Autodesk Inventor part; units mm, degrees
ref_plane "Work Plane2" through (17.8, 0, -35.7) normal (-1, 0, 0) x (0, 0, 1)
ref_plane "Work Plane3" through (20.6, 0, 2) normal (1, 0, 0) x (0, 0, -1)
ref_plane "YZ Plane" through (0, 0, 0) normal (1, 0, 0) x (0, 1, 0)
sketch "Sketch1" plane through (0, 0, 0) normal (0, 1, 0) x (-1, 0, 0)
  line L0 (0, 0) -> (-41.2, 0)
  line L1 (-41.2, 0) -> (-41.2, -33.7)
  line L2 (-41.2, -33.7) -> (0, -33.7)
  line L3 (0, -33.7) -> (0, 0)
  line L4 (2, 2) -> (-43.2, 2)
  line L5 (-43.2, 2) -> (-43.2, -35.7)
  line L6 (-43.2, -35.7) -> (2, -35.7)
  line L7 (2, -35.7) -> (2, 2)
  dimension "d0" = 33.7
  dimension "d1" = 41.2
  dimension "d2" = 2
  dimension "d3" = 2
  dimension "d4" = 2
  dimension "d5" = 2
extrude "Extrusion1" add sketch "Sketch1" along normal blind 2 contours L3 L2 L1 L0
extrude "Extrusion2" add sketch "Sketch1" along normal blind 120.5
sketch "Sketch2" plane through (41.2, 2, 0) normal (0, 0, -1) x (-1, 0, 0)
  line L0 (43.2, 118.5) -> (-2, 118.5)
  line L1 (36.2, 118.5) -> (31.2, 118.5)
  line L2 (31.2, 118.5) -> (31.2, 116.5)
  line L3 (31.2, 116.5) -> (36.2, 116.5)
  line L4 (36.2, 116.5) -> (36.2, 118.5)
  line L5 (41.2, 0) -> (41.2, 118.5)
  point P0 (41.2, -2)
  point P1 (31.2, 118.5)
  dimension "d10" = 5
  dimension "d11" = 2
  dimension "d12" = 5
sketch "Sketch3" plane through (41.2, 2, 0) normal (-1, 0, 0) x (0, 0, 1)
  point P0 (0, -2)
sketch "Sketch4" plane through (41.2, 2, 0) normal (-1, 0, 0) x (0, 0, 1)
  line L0 (2, 118.5) -> (-35.7, 118.5)
  line L1 (-5, 118.5) -> (-10, 118.5)
  line L2 (-10, 118.5) -> (-10, 116.5)
  line L3 (-10, 116.5) -> (-5, 116.5)
  line L4 (-5, 116.5) -> (-5, 118.5)
  line L5 (0, 0) -> (0, 118.5)
  point P0 (0, -2)
  dimension "d27" = 5
  dimension "d28" = 2
  dimension "d29" = 5
extrude "Extrusion4" add sketch "Sketch4" along normal blind 1.5
chamfer "Chamfer5" distance 0.75 distance2 1.5 1 edges at (39.7, 120.5, -7.5) measured on face at (39.7, 119.1667, -6.6667)
chamfer "Chamfer6" distance 0.75 distance2 1.5 1 edges at (39.7, 119.125, -10) measured on face at (39.7, 118.9167, -6.6667)
chamfer "Chamfer7" distance 0.75 distance2 1.5 1 edges at (39.7, 118.5, -7.1251) measured on face at (39.7, 119.3333, -7.8334)
chamfer "Chamfer8" distance 0.75 distance2 1.5 1 edges at (39.7, 119.5, -5) measured on face at (39.7, 119.5833, -6.4167)
sketch "Sketch5" plane through (0, 2, -33.7) normal (0, 0, 1) x (1, 0, 0)
  line L0 (0, 118.5) -> (41.2, 118.5)
  line L1 (36.2, 118.5) -> (31.2, 118.5)
  line L2 (31.2, 118.5) -> (31.2, 116.5)
  line L3 (31.2, 116.5) -> (36.2, 116.5)
  line L4 (36.2, 116.5) -> (36.2, 118.5)
  line L5 (41.2, 0) -> (41.2, 118.5)
  point P0 (0, -2)
  point P1 (31.2, 118.5)
  dimension "d45" = 5
  dimension "d46" = 2
  dimension "d47" = 5
extrude "Extrusion5" add sketch "Sketch5" along normal blind 1.5
chamfer "Chamfer9" distance 0.75 distance2 1.5 1 edges at (33.7, 120.5, -32.2) measured on face at (34.5333, 119.1667, -32.2)
chamfer "Chamfer10" distance 0.75 distance2 1.5 1 edges at (33.7, 118.5, -32.2) measured on face at (34.5333, 118.9167, -32.2)
chamfer "Chamfer11" distance 0.75 distance2 1.5 1 edges at (31.2, 119.4999, -32.2) measured on face at (34.5333, 119.4166, -32.2)
chamfer "Chamfer12" distance 0.75 distance2 1.5 1 edges at (36.2, 119.4999, -32.2) measured on face at (34.7833, 119.4166, -32.2)
ref_plane "Work Plane2" through (17.8, 0, -35.7) normal (-1, 0, 0) x (0, 0, 1)
ref_plane "Work Plane3" through (20.6, 0, 2) normal (1, 0, 0) x (0, 0, -1)
mirror "Mirror1" about plane through (20.6, 0, 2) normal (1, 0, 0) of "Extrusion5", "Extrusion4", "Chamfer5", "Chamfer8", "Chamfer7", "Chamfer9", "Chamfer11", "Chamfer10", "Chamfer12", "Chamfer6"
fillet "Fillet2" radius 3 3 edges at (-2, 0, -16.85) (20.6, 0, -35.7) (43.2, 0, -16.85)
fillet "Fillet3" radius 3 4 edges at (-1.1213, 0.8787, -34.8213) (-2, 61.75, -35.7) (42.3213, 0.8787, -34.8213) (43.2, 61.75, -35.7)
fillet "Fillet4" radius 3 2 edges at (0, 61.25, -33.7) (41.2, 61.25, -33.7)
sketch "Sketch10" plane through (-2, 120.5, 2) normal (0, 0, 1) x (1, 0, 0)
  line L0 (2, -24.4) -> (12, -24.4)
  line L1 (12, -24.4) -> (12, -34.4)
  line L2 (12, -34.4) -> (2, -34.4)
  line L3 (2, -34.4) -> (2, -24.4)
  line L4 (3, -120.5) -> (42.2, -120.5)
  line L5 (2, -118.5) -> (2, 0)
  line L6 (0, 0) -> (45.2, 0)
  point P0 (2, -120.5)
  dimension "d88" = 10
  dimension "d89" = 10
  dimension "d90" = 24.4
extrude "Extrusion10" cut sketch "Sketch10" against normal blind 10
sketch "Sketch11" plane through (-2, 120.5, 2) normal (0, 0, 1) x (1, 0, 0)
  line L0 (2, -108.5) -> (12, -108.5)
  line L1 (12, -108.5) -> (12, -118.5)
  line L2 (12, -118.5) -> (2, -118.5)
  line L3 (2, -118.5) -> (2, -108.5)
  line L4 (0, -117.5) -> (0, 0)
  line L5 (3, -120.5) -> (42.2, -120.5)
  point P0 (2, -120.5)
  dimension "d95" = 2
  dimension "d96" = 2
  dimension "d97" = 10
  dimension "d98" = 10
extrude "Extrusion11" cut sketch "Sketch11" against normal blind 10
sketch "Sketch12" plane through (43.2, 3, 2) normal (1, 0, 0) x (0, 0, -1)
  line L0 (26.35, 103.4808) -> (11.35, 107.5)
  arc A0 (25.4441, 100.1) -> (26.35, 103.4808) centre (25.8971, 101.7904) ccw
  line L1 (25.4441, 100.1) -> (10.4441, 104.1193)
  arc A1 (11.35, 107.5) -> (10.4441, 104.1193) centre (10.8971, 105.8096) ccw
  line L2 (0, 117.5) -> (34.7, 117.5)
  line L3 (0, 117.5) -> (37.7, 117.5)
  line L4 (10.4441, 104.1193) -> (10.4441, 103.1193)
  line L5 (37.7, 0) -> (37.7, 117.5)
  line L6 (26.35, 87.9641) -> (11.35, 91.9833)
  arc A2 (25.4441, 84.5834) -> (26.35, 87.9641) centre (25.8971, 86.2737) ccw
  line L7 (25.4441, 84.5834) -> (10.4441, 88.6026)
  arc A3 (11.35, 91.9833) -> (10.4441, 88.6026) centre (10.8971, 90.293) ccw
  line L8 (10.4441, 88.6026) -> (10.4441, 87.6026)
  line L9 (26.35, 72.4474) -> (11.35, 76.4667)
  arc A4 (25.4441, 69.0667) -> (26.35, 72.4474) centre (25.8971, 70.7571) ccw
  line L10 (25.4441, 69.0667) -> (10.4441, 73.0859)
  arc A5 (11.35, 76.4667) -> (10.4441, 73.0859) centre (10.8971, 74.7763) ccw
  line L11 (10.4441, 73.0859) -> (10.4441, 72.0859)
  line L12 (26.35, 56.9308) -> (11.35, 60.95)
  arc A6 (25.4441, 53.55) -> (26.35, 56.9308) centre (25.8971, 55.2404) ccw
  line L13 (25.4441, 53.55) -> (10.4441, 57.5692)
  arc A7 (11.35, 60.95) -> (10.4441, 57.5692) centre (10.8971, 59.2596) ccw
  line L14 (10.4441, 57.5692) -> (10.4441, 56.5692)
  line L15 (26.35, 41.4141) -> (11.35, 45.4333)
  arc A8 (25.4441, 38.0333) -> (26.35, 41.4141) centre (25.8971, 39.7237) ccw
  line L16 (25.4441, 38.0333) -> (10.4441, 42.0526)
  arc A9 (11.35, 45.4333) -> (10.4441, 42.0526) centre (10.8971, 43.7429) ccw
  line L17 (10.4441, 42.0526) -> (10.4441, 41.0526)
  line L18 (26.35, 25.8974) -> (11.35, 29.9166)
  arc A10 (25.4441, 22.5167) -> (26.35, 25.8974) centre (25.8971, 24.207) ccw
  line L19 (25.4441, 22.5167) -> (10.4441, 26.5359)
  arc A11 (11.35, 29.9166) -> (10.4441, 26.5359) centre (10.8971, 28.2263) ccw
  line L20 (10.4441, 26.5359) -> (10.4441, 25.5359)
  line L21 (26.35, 10.3807) -> (11.35, 14.4)
  arc A12 (25.4441, 7) -> (26.35, 10.3807) centre (25.8971, 8.6904) ccw
  line L22 (25.4441, 7) -> (10.4441, 11.0192)
  arc A13 (11.35, 14.4) -> (10.4441, 11.0192) centre (10.8971, 12.7096) ccw
  line L23 (10.4441, 11.0192) -> (10.4441, 10.0192)
  line L24 (0, -3) -> (34.7, -3)
  point P0 (18.85, 105.4904)
  point P1 (18.85, 117.5)
  point P2 (18.85, 89.9737)
  point P3 (18.85, 74.457)
  point P4 (18.85, 58.9404)
  point P5 (18.85, 43.4237)
  point P6 (18.85, 27.907)
  point P7 (18.85, 12.3904)
  dimension "d113" = 15
  dimension "d114" = 3.5
  dimension "d115" = 1
  dimension "d116" = 75
  dimension "d117" = 10
  dimension "d120" = 15.5167
  dimension "d125" = 10
extrude "Extrusion12" [suppressed]
sketch "Sketch13" plane through (-2, 3, 2) normal (-1, 0, 0) x (0, 0, 1)
  line L0 (-9.85, 103.4808) -> (-24.85, 107.5)
  arc A0 (-10.7559, 100.1) -> (-9.85, 103.4808) centre (-10.3029, 101.7904) ccw
  line L1 (-10.7559, 100.1) -> (-25.7559, 104.1193)
  arc A1 (-24.85, 107.5) -> (-25.7559, 104.1193) centre (-25.3029, 105.8096) ccw
  line L2 (-25.7559, 104.1193) -> (-25.7559, 103.1193)
  line L3 (0, -3) -> (0, 117.5)
  line L4 (-9.85, 87.9641) -> (-24.85, 91.9833)
  arc A2 (-10.7559, 84.5834) -> (-9.85, 87.9641) centre (-10.3029, 86.2737) ccw
  line L5 (-10.7559, 84.5834) -> (-25.7559, 88.6026)
  arc A3 (-24.85, 91.9833) -> (-25.7559, 88.6026) centre (-25.3029, 90.293) ccw
  line L6 (-25.7559, 88.6026) -> (-25.7559, 87.6026)
  line L7 (-9.85, 72.4474) -> (-24.85, 76.4667)
  arc A4 (-10.7559, 69.0667) -> (-9.85, 72.4474) centre (-10.3029, 70.7571) ccw
  line L8 (-10.7559, 69.0667) -> (-25.7559, 73.0859)
  arc A5 (-24.85, 76.4667) -> (-25.7559, 73.0859) centre (-25.3029, 74.7763) ccw
  line L9 (-25.7559, 73.0859) -> (-25.7559, 72.0859)
  line L10 (-9.85, 56.9308) -> (-24.85, 60.95)
  arc A6 (-10.7559, 53.55) -> (-9.85, 56.9308) centre (-10.3029, 55.2404) ccw
  line L11 (-10.7559, 53.55) -> (-25.7559, 57.5692)
  arc A7 (-24.85, 60.95) -> (-25.7559, 57.5692) centre (-25.3029, 59.2596) ccw
  line L12 (-25.7559, 57.5692) -> (-25.7559, 56.5692)
  line L13 (-9.85, 41.4141) -> (-24.85, 45.4333)
  arc A8 (-10.7559, 38.0333) -> (-9.85, 41.4141) centre (-10.3029, 39.7237) ccw
  line L14 (-10.7559, 38.0333) -> (-25.7559, 42.0526)
  arc A9 (-24.85, 45.4333) -> (-25.7559, 42.0526) centre (-25.3029, 43.7429) ccw
  line L15 (-25.7559, 42.0526) -> (-25.7559, 41.0526)
  line L16 (-9.85, 25.8974) -> (-24.85, 29.9166)
  arc A10 (-10.7559, 22.5167) -> (-9.85, 25.8974) centre (-10.3029, 24.207) ccw
  line L17 (-10.7559, 22.5167) -> (-25.7559, 26.5359)
  arc A11 (-24.85, 29.9166) -> (-25.7559, 26.5359) centre (-25.3029, 28.2263) ccw
  line L18 (-25.7559, 26.5359) -> (-25.7559, 25.5359)
  line L19 (-9.85, 10.3807) -> (-24.85, 14.4)
  arc A12 (-10.7559, 7) -> (-9.85, 10.3807) centre (-10.3029, 8.6904) ccw
  line L20 (-10.7559, 7) -> (-25.7559, 11.0192)
  arc A13 (-24.85, 14.4) -> (-25.7559, 11.0192) centre (-25.3029, 12.7096) ccw
  line L21 (-25.7559, 11.0192) -> (-25.7559, 10.0192)
  line L22 (0, 0) -> (0, -3)
  line L23 (-34.7, 117.5) -> (0, 117.5)
  line L24 (-34.7, -3) -> (0, -3)
  line L25 (-37.7, 0) -> (-37.7, 117.5)
  line L26 (0, 0) -> (0, 117.5)
  line L27 (-37.7, 117.5) -> (0, 117.5)
  point P0 (-17.35, 105.4904)
  point P1 (-17.35, 89.9737)
  point P2 (-17.35, 74.457)
  point P3 (-17.35, 58.9404)
  point P4 (-17.35, 43.4237)
  point P5 (-17.35, 27.907)
  point P6 (-17.35, 12.3904)
  point P7 (-17.35, 117.5)
  dimension "d132" = 15
  dimension "d133" = 3.5
  dimension "d134" = 1
  dimension "d135" = 75
  dimension "d137" = 15.5167
  dimension "d140" = 10
  dimension "d141" = 10
extrude "Extrusion13" [suppressed]
properties part number "Batterihållare 2"
Part model, mm, in its own coordinate system. A direction names the side the tool comes from. Give positions to 0.01 mm unless a question says otherwise; leave off trailing zeros. Loops run counter-clockwise (first coordinate to the right, second up) from the corner with the lowest first, then second, coordinate; pieces in that order, holes last. Notation, with made-up numbers: (53, 71.5) -> (59, 71.5) arc R19 cw to (59, 97.5) -> close; hole circle Ø2 at (88, -27). An arc over 180 degrees is marked (long way). Write each question's results on one line, items separated by ' | '. Start each with the question number.
Q1. Wall check: L1, parallel to Z at x = 9.5, y = 36.5; L2, parallel to X at y = 68.5, z = -23; L3, parallel to Y at x = 12, z = -6.5. Give the ranges that are in metal, low to high.
Q2. Pin check, flat tip, straight feed: P1, Ø10.5, axis at x = 11, z = -7.5, coming from the +Y side. Stop position of the tip, or through.
Q3. Band-saw the part on A-A on y = 26. List the corners of the cut face in (x, z), plus the area to 3 significant figures.
Q4. Pull direction X, two halves, no side cores. Call faces 1 (the face through (42.34, 0.9, -15.59)), 2 (the face through (40.34, 62.08, -32.8)), 3 (the face through (21, 61, -35.7)), 4 (the face through (-1.14, 0.9, -15.11)): +X half, -X half, draft (parallel to the pull), parting line (faces both ways), or undercut.
Q5. Band-saw the part on B-B on y = 8. List the corners of the cut face in (x, z), plus the area to 3 significant figures.
Q6. Which spindle directions (+Z, -Z, +X, -X, +Y, -Y) get a long thin tool onto all of the face, cutting with end or side? Do faces 5 (the face through (0.9, 62.08, -32.84)), 6 (the face through (42.3, 60.93, -34.84)), 7 (the face through (21, 60, -33.7)). Say none if no direction does.
Q7. Band-saw the part on D-D on x = 17. List the corners of the cut face in (y, z), plus the area to 3 significant figures.
Results are:
1) L1: z = -35.7 to -33.7, 0 to 2 | L2: x = -2 to 0, 41.2 to 43.2 | L3: y = 0 to 2
2) P1: stops at y = 2
3) outline: (-2, -32.7) arc R3 ccw to (1, -35.7) -> (40.2, -35.7) arc R3 ccw to (43.2, -32.7) -> (43.2, 2) -> (-2, 2) -> close; hole (0, -30.7) arc R3 ccw to (3, -33.7) -> (38.2, -33.7) arc R3 ccw to (41.2, -30.7) -> (41.2, 0) -> (0, 0) -> close | area: 316 mm²
4) face 1: +X half | face 2: undercut | face 3: draft | face 4: -X half
5) outline: (-2, -32.7) arc R3 ccw to (1, -35.7) -> (40.2, -35.7) arc R3 ccw to (43.2, -32.7) -> (43.2, 2) -> (10, 2) -> (10, 0) -> (41.2, 0) -> (41.2, -30.7) arc R3 cw to (38.2, -33.7) -> (3, -33.7) arc R3 cw to (0, -30.7) -> (0, 2) -> (-2, 2) -> close | area: 296 mm²
6) face 5: +Y | face 6: -Z, +X, +Y, -Y | face 7: none
7) outline: (0, -32.7) arc R3 ccw to (3, -35.7) -> (120.5, -35.7) -> (120.5, -33.7) -> (2, -33.7) -> (2, 0) -> (120.5, 0) -> (120.5, 2) -> (0, 2) -> close | area: 547 mm²
